Verification items for the finished model (mm, model axes). A direction names the side the tool comes from. Coordinates: 2 decimals unless noted, no trailing zeros. Write each loop counter-clockwise with the first axis right and the second up, starting at its lowest first coordinate (ties: lowest second). Pieces come first, ordered by that corner, then holes. Notation, with made-up numbers: (45, 78) - (76, 78) arc R28 cw to (76, 97) - close; hole circle Ø3 at (23, 22.5). An arc over 180 degrees is marked (long way). Answer as CSV lines item,"result". Start each with the question number.
```python
from build123d import *

# Parameters (mm, degrees)
F1_DEPTH = 6.35
F2_DEPTH = 3.175
F3_R     = 5
F4_R     = 3


# Not quite as in the source:
# - ends of sketch curves that miss each other by under 0.0002 mm in the source are joined
# - a feature names something its author has since deleted; it is built from what else it names


with BuildPart() as f1:
    # F0 (on Top) → F1 (new body)
    with BuildSketch(Plane.XY):
        Polygon((0, 12.50001), (0, 17.5), (-0.0375035219, 17.5), (-45.0252224641, 17.4621137515), (-54.9730516553, 2.5016534816), (-54.9460702886, -9.9983173986), (-45.0221895285, -17.4832638625), (-0.0259340823, -17.4999907076), (0, -17.5), (0, -12.50001), (-43.3485360617, -12.4839008237), (-49.9514424363, -7.508736751), (-49.9698707033, 1.0287403501), (-42.3475575474, 12.4643751943), align=None)
        Polygon((54.9832946886, 2.5222222222), (45, 17.5), (0, 17.5), (0, 12.50001), (42.3238055081, 12.50001), (49.9833046886, 1.0085855561), (49.9833046886, -7.4847291513), (43.3271563883, -12.50001), (0, -12.50001), (0, -17.5), (45, -17.5), (54.9832946886, -9.9777777778), align=None)
    extrude(amount=F1_DEPTH)

    # F0 (on Top) → F2 (join)
    with BuildSketch(Plane.XY):
        Polygon((0, -12.50001), (0, 12.50001), (-42.3475575474, 12.4643751943), (-49.9698707033, 1.0287403501), (-49.9514424363, -7.508736751), (-43.3485360617, -12.4839008237), align=None)
        Polygon((42.3238055081, 12.50001), (0, 12.50001), (0, -12.50001), (43.3271563883, -12.50001), (49.9833046886, -7.4847291513), (49.9833046886, 1.0085855561), align=None)
    extrude(amount=F2_DEPTH)

    # F3
    f3_edges = [f1.edges().sort_by_distance(p)[0] for p in [
        (-45.02219, -17.483264, 3.175),
        (-45.025222, 17.462114, 3.175),
        (45, 17.5, 3.175),
        (54.983295, 2.522222, 3.175),
        (54.983295, -9.977778, 3.175),
        (45, -17.5, 3.175),
        (-54.973052, 2.501653, 3.175),
        (-54.94607, -9.998317, 3.175),
    ]]
    fillet(f3_edges, radius=F3_R)

    # F4
    f4_edges = [f1.edges().sort_by_distance(p)[0] for p in [
        (-42.347558, 12.464375, 4.7625),
        (-49.969871, 1.02874, 4.7625),
        (-49.951442, -7.508737, 4.7625),
        (-43.348536, -12.483901, 4.7625),
        (43.327156, -12.50001, 4.7625),
        (49.983305, -7.484729, 4.7625),
        (49.983305, 1.008586, 4.7625),
        (42.323806, 12.50001, 4.7625),
    ]]
    fillet(f4_edges, radius=F4_R)


solid = f1.part
```
1. Scan lines: line 1 along X through (y, z) = (-2.5, 5.75); line 2 along Y through (x, z) = (-34.5, 5.5); line 3 along Z through (x, y) = (-44, -11) (3 decimals). Record each from-to range of solid material in increasing order. Write a range as from..to.
2. Cross-section at C-C (y = 8). Record the cut outline in (x, z) (3 decimals).
3. Cross-section at D-D (y = 13.5). Record the cut outline in (x, z), and give its area (3 significant figures).
4. Cross-section at B-B (x = 31). Record the cut outline in (y, z) (3 decimals).
5. Draft check along Y on faces 1 (the face through (-1, 0, 0)), 2 (the face through (-50.267, 9.579, 3.131)), 3 (the face through (43.29, -12.34, 4.78)), 4 (the face through (-54.44, -9.71, 3.22)). Enter one of: pulls with the +Y half, pulls with the -Y half, needs draft (parallel to the pull), parting line crosses it, or undercut.
6. Depth check by flat-ended pin: P1, Ø3.5, axis at x = -15.5, z = 4, coming from the +Y side; P2, Ø1.5, axis at y = 12, z = 4.5, coming from the +X side; P3, Ø3, axis at y = -9, z = 2.5, coming from the -X side. Enter the tip coordinate at first touch or a pass-through.
7. Access from +Z, -Z, +X, -X, +Y, -Y to the whole of each face (thin tool, end or side, straight path). Record for faces 5 (the face through (44.7, 16.9, 3.2)), 6 (the face through (-43.284, -12.333, 4.785)).
Completed:
1,line 1,"x = -54.96..-49.96, 49.98..54.98"
1,line 2,"y = -17.49..-12.49, 12.47..17.47"
1,line 3,"z = 0..3.175"
2,outline,"(-51.317, 0) - (51.332, 0) - (51.332, 6.35) - (45.323, 6.35) - (45.323, 3.175) - (-45.323, 3.175) - (-45.323, 6.35) - (-51.317, 6.35) - close"
3,outline,"(-47.66, 0) - (47.67, 0) - (47.67, 6.35) - (-47.66, 6.35) - close"
3,area,"605 mm2"
4,outline,"(-17.5, 0) - (17.5, 0) - (17.5, 6.35) - (12.5, 6.35) - (12.5, 3.175) - (-12.5, 3.175) - (-12.5, 6.35) - (-17.5, 6.35) - close"
5,face 1,"needs draft"
5,face 2,"pulls with the +Y half"
5,face 3,"undercut"
5,face 4,"pulls with the -Y half"
6,P1,"stops at y = 17.49"
6,P2,"stops at x = 49.17"
6,P3,"stops at x = -54.95"
7,face 5,"+Z, -Z, +X, +Y"
7,face 6,"+Z"
